from build123d import *

# Parameters (mm, degrees)
RESSALTO_EXTRUS_O1_DEPTH = 3


with BuildPart() as part:
    # Esboço1 → Ressalto-extrusão1 (new body)
    with BuildSketch(Plane(origin=(0, 0, 0), x_dir=(1, 0, 0), z_dir=(0, 1, 0))):
        with BuildLine():
            Line((37.16356961, 16.484544918), (0, 16.484544918))
            Line((0, 16.484544918), (0, 10.69506871))
            Line((0, 10.69506871), (-8.827691361, 10.69506871))
            Line((-8.827691361, 10.69506871), (-8.827691361, 16.484544918))
            Line((-8.827691361, 16.484544918), (-44.03643039, 16.484544918))
            ThreePointArc((-44.03643039, 16.484544918), (-46.711254325, 16.041404638), (-47.93643039, 13.622727314))
            Line((-47.93643039, 13.622727314), (-47.93643039, 4.0833353))
            Line((-47.93643039, 4.0833353), (-47.93643039, -9.9166647))
            ThreePointArc((-47.93643039, -9.9166647), (-46.764857515, -12.745091825), (-43.93643039, -13.9166647))
            Line((-43.93643039, -13.9166647), (37.06356961, -13.9166647))
            ThreePointArc((37.06356961, -13.9166647), (39.891996735, -12.745091825), (41.06356961, -9.9166647))
            Line((41.06356961, -9.9166647), (41.06356961, 4.0833353))
            Line((41.06356961, 4.0833353), (41.06356961, 13.622727314))
            ThreePointArc((41.06356961, 13.622727314), (39.838393545, 16.041404638), (37.16356961, 16.484544918))
        make_face()
    extrude(amount=RESSALTO_EXTRUS_O1_DEPTH)


solid = part.part
CAD build for the part. Positions are in the model's coordinates, mm. A direction names the side the tool comes from. Give positions to 0.01 mm unless a question says otherwise; leave off trailing zeros. Write each loop counter-clockwise with the first axis right and the second up, starting at its lowest first coordinate (ties: lowest second). Pieces come first, ordered by that corner, then holes. Notation, with made-up numbers: (84, 64) - (140, 64) arc R13 ccw to (140, 69) - close; hole circle Ø7 at (14, 67.25). An arc over 180 degrees is marked (long way). Answer as CSV lines item,"result".
Q1. Drill centre lines: line 1 (X direction, y = 0.7, z = -13.5); line 2 (Z direction, x = 21.5, y = 2.85); line 3 (Z direction, x = -7, y = 2.05). Where is each one in solid material? Low to high. Write a range as from..to.
Result set:
line 1,"-47.94..-8.83, 0..41.06"
line 2,"-16.48..13.92"
line 3,"-10.7..13.92"
Q2. Band-saw the part on A-A (y = 1.5). Give the cut face in (x, z), and give its area (3 significant figures).
Result set:
outline,"(-47.94, -13.62) arc R3 ccw to (-44.04, -16.48) - (-8.83, -16.48) - (-8.83, -10.7) - (0, -10.7) - (0, -16.48) - (37.16, -16.48) arc R3 ccw to (41.06, -13.62) - (41.06, 9.92) arc R4 ccw to (37.06, 13.92) - (-43.94, 13.92) arc R4 ccw to (-47.94, 9.92) - close"
area,"2,640 mm²"
Q3. 3-axis set-ups, long thin cutter, end or side, ignore diameter. For faces 1 (the face through (0, 1, -14)), 2 (the face through (-4, 0, -2)): which of +Z, -Z, +X, -X, +Y, -Y reach the whole face in a straight line?
Result set:
face 1,"-Z, +Y, -Y"
face 2,"+Z, -Z, +X, -X, -Y"
Q4. Flat gauge pins, fed straight in: pin 1 Ø1.5 at (y, z) = (1, -14.5) entering from -X; pin 2 Ø1.5 at (x, y) = (-29.5, 2) entering from -Z; pin 3 Ø1.5 at (y, z) = (1, -15) entering from +X. Where does each tip first touch, or does it go through?
Result set:
pin 1,"x = -47.93"
pin 2,"z = -16.48"
pin 3,"x = 41"
Q5. Pull direction X, two halves, no side cores. Call faces 3 (the face through (-4, 1, 13.917)), 4 (the face through (-8.828, 1, -14)), 5 (the face through (-46.8, 1.48, 12.71)), 6 (the face through (41.064, 1, -2)): released by +X, released by -X, zero draft, split by the parting line, or undercut.
Result set:
face 3,"zero draft"
face 4,"undercut"
face 5,"released by -X"
face 6,"released by +X"
Q6. Band-saw the part on B-B (x = -8). Give the cut face in (y, z).
Result set:
outline,"(0, -10.7) - (3, -10.7) - (3, 13.92) - (0, 13.92) - close"
Q7. Band-saw the part on C-C (z = 12.5). Give the cut face in (x, y), and give its area (3 significant figures).
Result set:
outline,"(-46.99, 0) - (40.12, 0) - (40.12, 3) - (-46.99, 3) - close"
area,"261 mm²"
